Geometry check sheet. Reference: the model listing, model coordinates, mm. Give positions to 0.01 mm unless a question says otherwise; leave off trailing zeros. Write each loop counter-clockwise with the first axis right and the second up, starting at its lowest first coordinate (ties: lowest second). Pieces come first, ordered by that corner, then holes. Notation, with made-up numbers: (0, 55) - (27, 55) arc R9 ccw to (27, 68) - close; hole circle Ø3 at (57.25, 62.5). An arc over 180 degrees is marked (long way). Use a Markdown table: item, result.
```python
from build123d import *

# Parameters (mm, degrees)
EXTRUDE_1_DEPTH     = 3
SKETCH_2_R          = 1.5
CUT_EXTRUDE_1_DEPTH = 3


with BuildPart() as part:
    # 草图1 → 凸台-拉伸1 (new body)
    with BuildSketch(Plane.XY):
        with BuildLine():
            Line((-45, 24), (45, 24))
            ThreePointArc((45, 24), (48.535533906, 22.535533906), (50, 19))
            Line((50, 19), (50, -19))
            ThreePointArc((50, -19), (48.535533906, -22.535533906), (45, -24))
            Line((45, -24), (-45, -24))
            ThreePointArc((-45, -24), (-48.535533906, -22.535533906), (-50, -19))
            Line((-50, -19), (-50, 19))
            ThreePointArc((-50, 19), (-48.535533906, 22.535533906), (-45, 24))
        make_face()
    extrude(amount=EXTRUDE_1_DEPTH)

    # 草图2 → 切除-拉伸1 (cut)
    with BuildSketch(Plane.XY.offset(3)):
        with Locations((-46, 20)):
            Circle(SKETCH_2_R)
        with Locations((46, 20)):
            Circle(SKETCH_2_R)
        with Locations((-46, -20)):
            Circle(SKETCH_2_R)
        with Locations((46, -20)):
            Circle(SKETCH_2_R)
    extrude(amount=-CUT_EXTRUDE_1_DEPTH, mode=Mode.SUBTRACT)


solid = part.part
```
1) Section check A-A on y = -20. Record the boundary of the cut face in (x, z), then the cut area to 3 significant figures.
Working result:
| item | result |
|---|---|
| outline | (-49.9, 0) - (-47.5, 0) - (-47.5, 3) - (-49.9, 3) - close; (-44.5, 0) - (44.5, 0) - (44.5, 3) - (-44.5, 3) - close; (47.5, 0) - (49.9, 0) - (49.9, 3) - (47.5, 3) - close |
| area | 281 mm² |
2) Section check B-B on x = -46. Record the boundary of the cut face in (y, z).
Working result:
| item | result |
|---|---|
| outline | (-23.9, 0) - (-21.5, 0) - (-21.5, 3) - (-23.9, 3) - close; (-18.5, 0) - (18.5, 0) - (18.5, 3) - (-18.5, 3) - close; (21.5, 0) - (23.9, 0) - (23.9, 3) - (21.5, 3) - close |
3) Mould release check, pull along Y, two halves, no side actions. Record for faces 1 (the cylindrical face through (-48, -23, 1)), 2 (the flat face through (-1, 24, 1)), 3 (the cylindrical face through (44.5, -19.93, 1.52)): pulls with the +Y half, pulls with the -Y half, needs draft (parallel to the pull), parting line crosses it, or undercut.
Working result:
| item | result |
|---|---|
| face 1 | pulls with the -Y half |
| face 2 | pulls with the +Y half |
| face 3 | undercut |
4) Material ranges on L1, parallel to X at y = -21, z = 2.65; L2, parallel to Y at x = -46, z = 2.3, recorded low to high. Write a range as from..to.
Working result:
| item | result |
|---|---|
| L1 | x = -49.58..-47.12, -44.88..44.88, 47.12..49.58 |
| L2 | y = -23.9..-21.5, -18.5..18.5, 21.5..23.9 |
